from build123d import *

# Parameters (mm, degrees)
F0_W     = 25.4
F0_H     = 15.759564
F1_DEPTH = 6.35
F2_DEPTH = 3.81


with BuildPart() as f1:
    # F0 (on Top) → F1 (new body)
    with BuildSketch(Plane.XY):
        Rectangle(F0_W, F0_H)
        Polygon((-10.654746, -4.793949), (-10.654746, 4.793949), (-1.625014, 0), align=None, mode=Mode.SUBTRACT)
        Polygon((9.029732, -5.65668), (-9.029732, -5.65668), (0, -0.862732), align=None, mode=Mode.SUBTRACT)
        Polygon((0, 0.862732), (-9.029732, 5.65668), (9.029732, 5.65668), align=None, mode=Mode.SUBTRACT)
        Polygon((1.625014, 0), (10.654746, 4.793949), (10.654746, -4.793949), align=None, mode=Mode.SUBTRACT)
    extrude(amount=F1_DEPTH)

    # F0 (on Top) → F2 (join)
    with BuildSketch(Plane.XY):
        Polygon((9.029732, 5.65668), (-9.029732, 5.65668), (0, 0.862732), align=None)
        Polygon((-1.625014, 0), (-10.654746, 4.793949), (-10.654746, -4.793949), align=None)
        Polygon((0, -0.862732), (-9.029732, -5.65668), (9.029732, -5.65668), align=None)
        Polygon((10.654746, -4.793949), (10.654746, 4.793949), (1.625014, 0), align=None)
    extrude(amount=F2_DEPTH)


solid = f1.part
Source: CAD feature listing. Evaluate the final solid. Frame: model axes, mm. A direction names the side the tool comes from. Give positions to 0.01 mm unless a question says otherwise; leave off trailing zeros. Write each loop counter-clockwise with the first axis right and the second up, starting at its lowest first coordinate (ties: lowest second). Pieces come first, ordered by that corner, then holes. Notation, with made-up numbers: (1.5, 26.25) -> (40.5, 26.25) arc R27 cw to (40.5, 49.25) -> close; hole circle Ø6 at (-7.75, 33.25). An arc over 180 degrees is marked (long way). Write item = value, one per line.
Q1. Cut plane B-B on x = 2.5. Return loops of the section in (y, z).
Here are the results:
outline = (-7.88, 0) -> (7.88, 0) -> (7.88, 6.35) -> (5.66, 6.35) -> (5.66, 3.81) -> (2.19, 3.81) -> (2.19, 6.35) -> (0.46, 6.35) -> (0.46, 3.81) -> (-0.46, 3.81) -> (-0.46, 6.35) -> (-2.19, 6.35) -> (-2.19, 3.81) -> (-5.66, 3.81) -> (-5.66, 6.35) -> (-7.88, 6.35) -> close
Q2. Reachability of faces 1 (the face through (0, 0, 6.35)), 2 (the face through (0, -4, 3.81)) from +Z, -Z, +X, -X, +Y, -Y: full face, straight path, thin tool, end or side. Return the list, or none.
Here are the results:
face_1 = +Z, +X, -X, +Y, -Y
face_2 = +Z
Q3. Cut plane A-A on z = 4.75. Return loops of the section in (x, y).
Here are the results:
outline = (-12.7, -7.88) -> (12.7, -7.88) -> (12.7, 7.88) -> (-12.7, 7.88) -> close; hole (-10.65, -4.79) -> (-1.63, 0) -> (-10.65, 4.79) -> close; hole (-9.03, -5.66) -> (9.03, -5.66) -> (0, -0.86) -> close; hole (-9.03, 5.66) -> (0, 0.86) -> (9.03, 5.66) -> close; hole (1.63, 0) -> (10.65, -4.79) -> (10.65, 4.79) -> close
Q4. First-contact query: pin 1 (2.5 mm diameter, centred on x = -8.5, y = -2, fed in from +Z). Flat tip, straight axial feed; report the tip coordinate or a pass-through.
Here are the results:
pin_1 = 3.81
Q5. Cut plane C-C on y = -5.25. Return loops of the section in (x, z), then the cut area to 3 significant figures.
Here are the results:
outline = (-12.7, 0) -> (12.7, 0) -> (12.7, 6.35) -> (8.26, 6.35) -> (8.26, 3.81) -> (-8.26, 3.81) -> (-8.26, 6.35) -> (-12.7, 6.35) -> close
area = 119 mm²
Q6. Mould query, pull axis Y, two halves, no side actions, for faces 3 (the face through (0, 4, 3.81)), 4 (the face through (12.7, 0, 3)), 5 (the face through (0, -7.88, 3)). Classes: +Y half, -Y half, draft (parallel to the pull), parting line (faces both ways), or undercut.
Here are the results:
face_3 = undercut
face_4 = draft
face_5 = -Y half
Q7. Line query: line 1 (Y direction, x = 8.5, z = 5); line 2 (Y direction, x = -7.25, z = 5.75); line 3 (Y direction, x = 1.25, z = 4.75). Output: solid intervals per line, ascending. Write a range as from..to.
Here are the results:
line_1 = -7.88..-5.66, -5.38..-3.65, 3.65..5.38, 5.66..7.88
line_2 = -7.88..-5.66, -4.71..-2.99, 2.99..4.71, 5.66..7.88
line_3 = -7.88..-5.66, -1.53..1.53, 5.66..7.88
Q8. Cut plane D-D on x = -0.25. Return loops of the section in (y, z).
Here are the results:
outline = (-7.88, 0) -> (7.88, 0) -> (7.88, 6.35) -> (5.66, 6.35) -> (5.66, 3.81) -> (1, 3.81) -> (1, 6.35) -> (-1, 6.35) -> (-1, 3.81) -> (-5.66, 3.81) -> (-5.66, 6.35) -> (-7.88, 6.35) -> close
